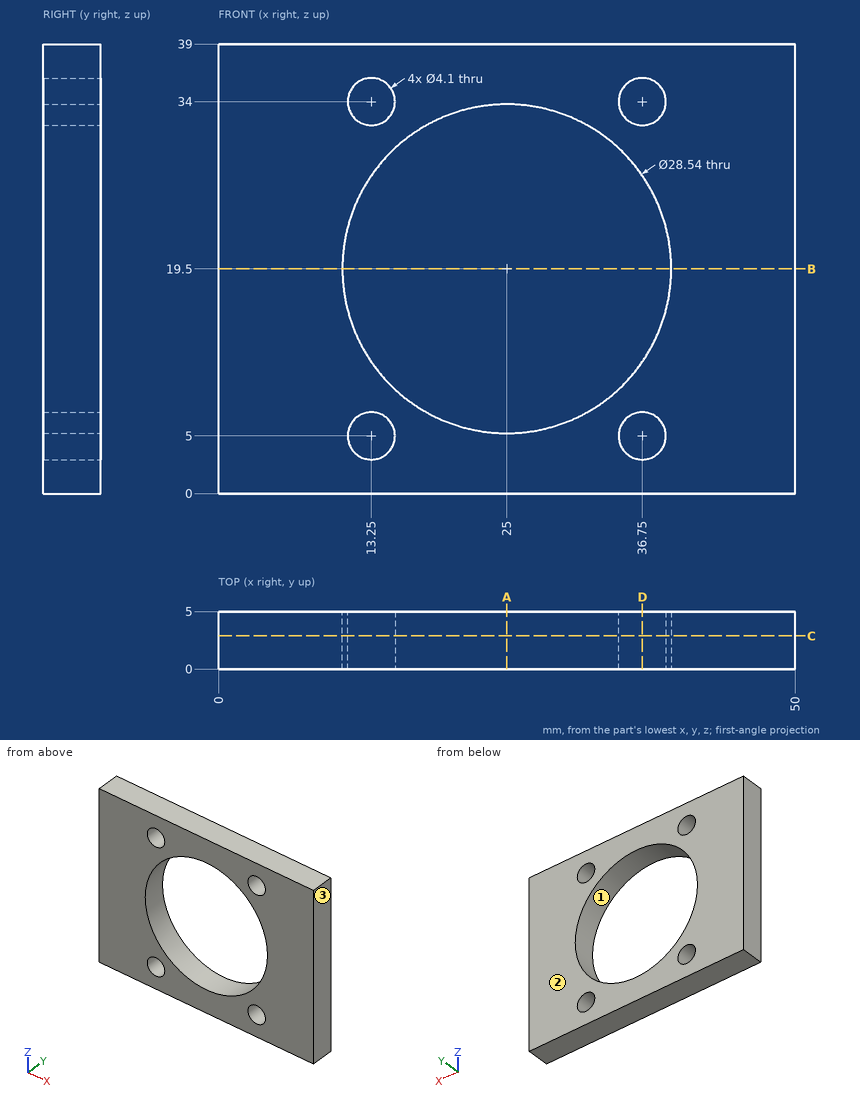
Input: dimensioned drawing with shaded views. Units: mm. Origin: part minimum x, y, z. Round coordinates to 2 decimals unless told otherwise and drop trailing zeros. Loops run counter-clockwise (first coordinate to the right, second up) from the corner with the lowest first, then second, coordinate; pieces in that order, holes last.
1) Pin query (flat end, axial travel): pin 1 (1 mm diameter, centred on y = 3.5, z = 17, fed in from -X). Return the tip coordinate at first contact, or that it passes through.
Ans:
pin 1: stops at x = 0
2) Section query A-A on x = 25. Return the cut outline in (y, z), plus the area to 3 significant figures.
Ans:
outline: (0, 0) - (5, 0) - (5, 5.23) - (0, 5.23) - close; (0, 33.77) - (5, 33.77) - (5, 39) - (0, 39) - close
area: 52.3 mm2
3) Section query D-D on x = 36.75. Return the cut outline in (y, z), plus the area to 3 significant figures.
Ans:
outline: (0, 0) - (5, 0) - (5, 2.95) - (0, 2.95) - close; (0, 7.05) - (5, 7.05) - (5, 11.4) - (0, 11.4) - close; (0, 27.6) - (5, 27.6) - (5, 31.95) - (0, 31.95) - close; (0, 36.05) - (5, 36.05) - (5, 39) - (0, 39) - close
area: 73.0 mm2
4) Section query B-B on z = 19.5. Return the cut outline in (x, y).
Ans:
outline: (0, 0) - (10.73, 0) - (10.73, 5) - (0, 5) - close; (39.27, 0) - (50, 0) - (50, 5) - (39.27, 5) - close
5) Pull-direction query (X, two-part tool) for the marked faces 1, 2 and 3; classes: released by +X, released by -X, zero draft, split by the parting line, or undercut.
Ans:
face 1: undercut
face 2: zero draft
face 3: released by +X
6) Material intervals for line 1 (Z direction, x = 35, y = 0.8); line 2 (Z direction, x = 36.75, y = 1.8); line 3 (Z direction, x = 25, y = 4), sorted ascending.
Ans:
line 1: z = 0 to 3.93, 6.07 to 9.32, 29.68 to 32.93, 35.07 to 39
line 2: z = 0 to 2.95, 7.05 to 11.4, 27.6 to 31.95, 36.05 to 39
line 3: z = 0 to 5.23, 33.77 to 39
7) Section query C-C on y = 2.9. Return the cut outline in (x, z).
Ans:
outline: (0, 0) - (50, 0) - (50, 39) - (0, 39) - close; hole circle Ø28.54 at (25, 19.5); hole circle Ø4.1 at (13.25, 5); hole circle Ø4.1 at (13.25, 34); hole circle Ø4.1 at (36.75, 5); hole circle Ø4.1 at (36.75, 34)
